from build123d import *

# Parameters (mm, degrees)
EXTRUSION1_DEPTH = 2.5
SKETCH2_R        = 3.75
EXTRUSION2_DEPTH = 1
HOLE1_D          = 4.917
FILLET1_R        = 0.5


with BuildPart() as part:
    # Sketch1 → Extrusion1 (new body)
    with BuildSketch(Plane.XY):
        with BuildLine():
            Line((-10.25, -5.6), (10.25, -5.6))
            ThreePointArc((10.25, -5.6), (12.6, 0), (10.25, 5.6))
            Line((10.25, 5.6), (-10.25, 5.6))
            ThreePointArc((-10.25, 5.6), (-12.6, 0), (-10.25, -5.6))
        make_face()
    extrude(amount=EXTRUSION1_DEPTH)

    # Sketch2 → Extrusion2 (add)
    with BuildSketch(Plane.XY.offset(2.5)):
        Circle(SKETCH2_R)
    extrude(amount=EXTRUSION2_DEPTH)

    # Hole1 (through all)
    with Locations(Plane.XY.offset(3.5)):
        with Locations((0, 0)):
            Hole(HOLE1_D / 2)

    # Fillet1
    fillet1_edges = [part.edges().sort_by_distance(p)[0] for p in [
        (12.6, 0, 2.5),
        (0, 5.6, 2.5),
        (-3.75, 0, 3.5),
        (-12.6, 0, 2.5),
        (0, -5.6, 2.5),
    ]]
    fillet(fillet1_edges, radius=FILLET1_R)


solid = part.part
Geometry check sheet. Reference: the model listing, model coordinates, mm. A direction names the side the tool comes from. Round coordinates to 2 decimals unless told otherwise and drop trailing zeros. Order: outer loops, then holes, each group sorted by start corner. A loop starts at its lowest first (then second) coordinate and runs counter-clockwise, first axis right, second up. Notation, with made-up numbers: M 13.25,42.5 L 46.25,42.5 A7 cw 46.25,52.5 Z; hole C 0,28 d3. An arc over 180 degrees is marked long. Write each question's results on one line, items separated by ' | '. Start each with the question number.
1. Draft check along X on faces 1 (the face through (-12.6, 0.1, 1)), 2 (the face through (-2.345, 0.738, 1.726)), 3 (the face through (0, 3, 0)). Enter one of: pulls with the +X half, pulls with the -X half, needs draft (parallel to the pull), parting line crosses it, or undercut.
2. Cross-section at A-A on y = 0. Record the boundary of the cut face in (x, z).
3. Set-up check for faces 4 (the face through (-3.746, 0.165, 2.746)), 5 (the face through (-2, 2, 3.5)): record each of +Z, -Z, +X, -X, +Y, -Y from which the full face is reachable in a straight line by a thin tool's end or side.
4. Go/stop test with flat-tipped pins: P1, Ø2, axis at y = 3, z = 2, coming from the +X side; P2, Ø1, axis at y = 1.5, z = 2, coming from the +X side. Record where each tip stops, or that it passes through.
5. Cross-section at D-D on x = 4.25. Record the boundary of the cut face in (y, z).
6. Material ranges on L1, parallel to Y at x = 0, z = 1.85; L2, parallel to Y at x = 0, z = 2.55; L3, parallel to Z at x = 8.5, y = 4, recorded low to high. Write a range as from..to.
7. Cross-section at C-C on x = 0. Record the boundary of the cut face in (y, z), plus the area to 3 significant figures.
8. Cross-section at B-B on z = 1.2. Record the boundary of the cut face in (x, y), plus the area to 3 significant figures.
Resolved:
1) face 1: pulls with the -X half | face 2: undercut | face 3: needs draft
2) outline: M -12.6,0 L -2.46,0 L -2.46,3.5 L -3.25,3.5 A0.5 ccw -3.75,3 L -3.75,2.5 L -12.1,2.5 A0.5 ccw -12.6,2 Z; M 2.46,0 L 12.6,0 L 12.6,2 A0.5 ccw 12.1,2.5 L 3.75,2.5 L 3.75,3 A0.5 ccw 3.25,3.5 L 2.46,3.5 Z
3) face 4: +Z | face 5: +Z, +X, -X, +Y, -Y
4) P1: x = 12.34 | P2: x = 12.54
5) outline: M -5.6,0 L 5.6,0 L 5.6,2 A0.5 ccw 5.1,2.5 L -5.1,2.5 A0.5 ccw -5.6,2 Z
6) L1: -5.6..-2.46, 2.46..5.6 | L2: -3.75..-2.46, 2.46..3.75 | L3: 0..2.5
7) outline: M -5.6,0 L -2.46,0 L -2.46,3.5 L -3.25,3.5 A0.5 ccw -3.75,3 L -3.75,2.5 L -5.1,2.5 A0.5 ccw -5.6,2 Z; M 2.46,0 L 5.6,0 L 5.6,2 A0.5 ccw 5.1,2.5 L 3.75,2.5 L 3.75,3 A0.5 ccw 3.25,3.5 L 2.46,3.5 Z | area: 18.1 mm2
8) outline: M -10.25,-5.6 L 10.25,-5.6 A7.85 ccw 10.25,5.6 L -10.25,5.6 A7.85 ccw Z; hole C 0,0 d4.92 | area: 247 mm2
